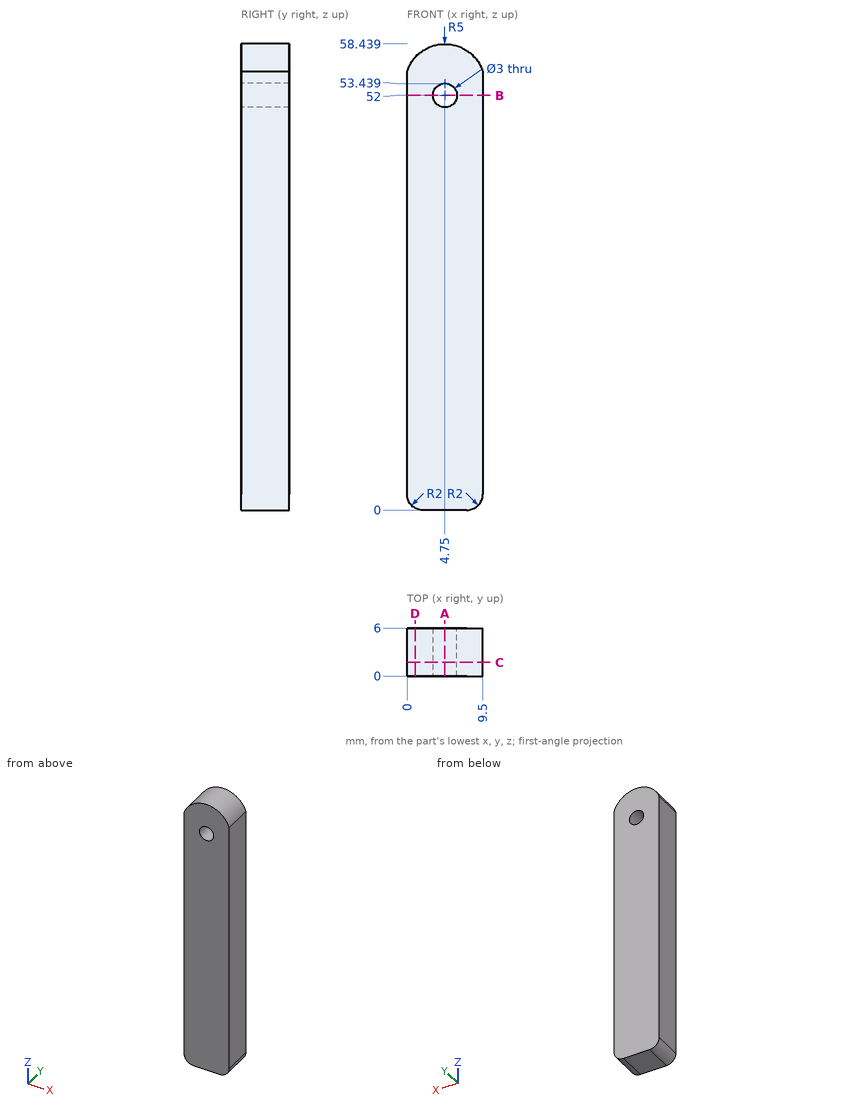
Source: three-view drawing plus pictorial views. Frame: mm from the lowest corner of the part. Give positions to 0.01 mm unless a question says otherwise; leave off trailing zeros. Write each loop counter-clockwise with the first axis right and the second up, starting at its lowest first coordinate (ties: lowest second). Pieces come first, ordered by that corner, then holes.
(1) Cut plane D-D, the plane x = 1. Return loops of the section in (y, z).
(2) Cut plane B-B, the plane z = 52. Return loops of the section in (x, y).
(3) Cut plane C-C, the plane y = 1.7. Return loops of the section in (x, z), then the cut area to 3 significant figures.
(4) Ray query, line 1 (Z direction, x = 4.75, y = 3.8); line 2 (X direction, y = 3.25, z = 52); line 3 (X direction, y = 5.7, z = 53). Return the intervals inside material, ascending.
(5) Cut plane A-A, the plane x = 4.75. Return loops of the section in (y, z).
Values follow:
1. outline: (0, 0.27) - (6, 0.27) - (6, 56.75) - (0, 56.75) - close
2. outline: (0, 0) - (3.25, 0) - (3.25, 6) - (0, 6) - close; (6.25, 0) - (9.5, 0) - (9.5, 6) - (6.25, 6) - close
3. outline: (0, 2) arc R2 ccw to (2, 0) - (7.5, 0) arc R2 ccw to (9.5, 2) - (9.5, 55) arc R5 ccw to (0, 55) - close; hole circle Ø3 at (4.75, 52)
3. area: 538 mm2
4. line 1: z = 0 to 50.5, 53.5 to 58.44
4. line 2: x = 0 to 3.25, 6.25 to 9.5
4. line 3: x = 0 to 3.63, 5.87 to 9.5
5. outline: (0, 0) - (6, 0) - (6, 50.5) - (0, 50.5) - close; (0, 53.5) - (6, 53.5) - (6, 58.44) - (0, 58.44) - close
